```python
from build123d import *

# Parameters (mm, degrees)
FILLET1_R           = 1.25
BOSS_EXTRUDE1_REACH = 17.399
SKETCH8_R           = 2.8
SKETCH12_R          = 2.4
CUT_EXTRUDE8_DEPTH  = 6


with BuildPart() as part:
    # Sketch6 → Loft2 section 0
    with BuildSketch(Plane(origin=(0, 9.3, 0), x_dir=(1, 0, 0), z_dir=(0, 1, 0))):
        with BuildLine():
            Line((-7.324, 7.255), (7.324, 7.255))
            Line((7.324, 7.255), (7.324, -7.255))
            Line((7.324, -7.255), (-7.324, -7.255))
            Line((-7.324, -7.255), (-7.324, 7.255))
        make_face()
    # Sketch5 → Loft2 section 1
    with BuildSketch(Plane(origin=(0, 0, 0), x_dir=(1, 0, 0), z_dir=(0, 1, 0))):
        with BuildLine():
            Line((-8.9845, 8.9845), (8.9845, 8.9845))
            Line((8.9845, 8.9845), (8.9845, -8.9845))
            Line((8.9845, -8.9845), (-8.9845, -8.9845))
            Line((-8.9845, -8.9845), (-8.9845, 8.9845))
        make_face()
    loft()

    # Fillet1
    fillet1_edges = [part.edges().sort_by_distance(p)[0] for p in [
        (8.15425, 4.65, -8.11975),
        (8.15425, 4.65, 8.11975),
        (-8.15425, 4.65, -8.11975),
        (-8.15425, 4.65, 8.11975),
    ]]
    fillet(fillet1_edges, radius=FILLET1_R)

    # Shell1: read off the stored shape, not the designer's step
    # Shell1: loft between two sections, ruled curve by curve
    shell1_from = [
        Edge.make_line((-7.714731612, 0, -7.713068719), (7.714731612, 0, -7.713068719)),
        Edge.make_line((-7.714731612, 0, 7.713068719), (-7.714731612, 0, -7.713068719)),
        Edge.make_line((7.714731612, 0, 7.713068719), (7.714731612, 0, -7.713068719)),
        Edge.make_line((-7.714731612, 0, 7.713068719), (7.714731612, 0, 7.713068719)),
    ]
    shell1_to = [
        Edge.make_line((-6.277417095, 8.05, -6.216028397), (6.277417095, 8.05, -6.216028397)),
        Edge.make_line((-6.277417095, 8.05, 6.216028397), (-6.277417095, 8.05, -6.216028397)),
        Edge.make_line((6.277417095, 8.05, 6.216028397), (6.277417095, 8.05, -6.216028397)),
        Edge.make_line((-6.277417095, 8.05, 6.216028397), (6.277417095, 8.05, 6.216028397)),
    ]
    shell1 = Solid(Shell([*[Face.make_surface_from_curves(shell1_from[k], shell1_to[k]) for k in range(4)], Face(Wire(shell1_from)), Face(Wire(shell1_to))]))
    add(shell1, mode=Mode.SUBTRACT)

    # Sketch8 → Boss-Extrude1 (add, up to next)
    with BuildSketch(Plane(origin=(0, 0.6, 0), x_dir=(1, 0, 0), z_dir=(0, 1, 0)), mode=Mode.PRIVATE) as boss_extrude1_sk1:
        with Locations(Location((0, 0, 0), (0, 0, 270))):
            Circle(SKETCH8_R)
    boss_extrude1_tool1 = extrude(boss_extrude1_sk1.sketch, amount=BOSS_EXTRUDE1_REACH, mode=Mode.PRIVATE) - part.part
    add(boss_extrude1_tool1.solids().sort_by_distance((0, 0.6, 0))[0])

    # Sketch12 → Cut-Extrude8 (cut)
    with BuildSketch(Plane(origin=(0, 0.6, 0), x_dir=(1, 0, 0), z_dir=(0, 1, 0))):
        with Locations(Location((0, 0, 0), (0, 0, 270))):
            Circle(SKETCH12_R)
    extrude(amount=CUT_EXTRUDE8_DEPTH, mode=Mode.SUBTRACT)


solid = part.part
```
Geometry: final body of the model. Coordinates: model frame, mm. A direction names the side the tool comes from. Round coordinates to 2 decimals unless told otherwise and drop trailing zeros.
Item 1: Mould query, pull axis X, two halves, no side actions, for faces 3 (the face through (0.1, 4.3, -2.8)), 4 (the face through (0, 0, -8)). Classes: +X half, -X half, draft (parallel to the pull), parting line (faces both ways), or undercut.
Item 2: Section query A-A (y = 7.25). Give the number of separate pieces and of enclosed holes in the cut face, plus the area to 3 significant figures.
Item 3: Set-up query: faces 1 (the face through (0, 8.05, 3)), 2 (the face through (0, 9.3, 0)). Return all of +Z, -Z, +X, -X, +Y, -Y with unobstructed straight access to the full face (end or side cutting, diameter ignored); none if empty.
Item 4: Material intervals for L1, parallel to X at y = 4.45, z = 0; L2, parallel to X at y = 3.1, z = 0; L3, parallel to Y at x = 1.5, z = 4.75, sorted ascending.
Item 5: Pin query (flat end, axial travel): P1, Ø2, axis at x = 1.5, y = 2, coming from the -Z side; P2, Ø4, axis at x = -5.5, y = 3.5, coming from the -Z side; P3, Ø2.5, axis at x = -0.5, z = -0.5, coming from the -Y side. Return the tip coordinate at first contact, or that it passes through.
Completed:
1. face 3: undercut
1. face 4: draft
2. separate pieces: 2
2. enclosed holes: 1
2. area: 94.8 mm2
3. face 1: -Y
3. face 2: +Z, -Z, +X, -X, +Y
4. L1: x = -8.19 to -6.92, -2.8 to -2.4, 2.4 to 2.8, 6.92 to 8.19
4. L2: x = -8.43 to -7.16, -2.8 to -2.4, 2.4 to 2.8, 7.16 to 8.43
4. L3: y = 8.05 to 9.3
5. P1: stops at z = -8.8
5. P2: stops at z = -8.71
5. P3: stops at y = 6.6
